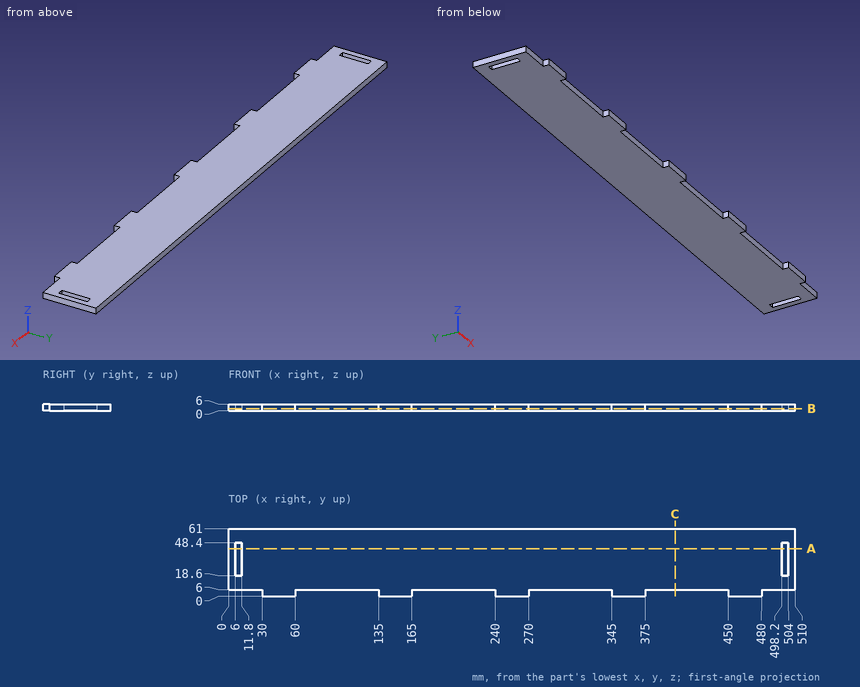
Could you check a few things on this drawing? It's one solid part, dimensions in mm from its lowest x, y, z. Round coordinates to 2 decimals unless told otherwise and drop trailing zeros. Loops run counter-clockwise (first coordinate to the right, second up) from the corner with the lowest first, then second, coordinate; pieces in that order, holes last. Notation, with made-up numbers: (16, -34.5) -> (47, -34.5) arc R28 cw to (47, -6.5) -> close; hole circle Ø1 at (45.5, 68.5). An arc over 180 degrees is marked (long way). One line per item, written item: value. Start each with the question number.
1. If we section it at B-B, the plane z = 1.75: Give the number of separate pieces and of enclosed holes in the cut face, then the cut area to 3 significant figures.
2. If I drill on probe 1 along X at (y, z) = (30, 2.5); probe 2 along Y at (x, z) = (306, 2.65), over which ranges is the centre line in solid material (lowest first)?
3. If we section it at A-A, the plane y = 43: Write out the boundary of the cut face in (x, z).
4. For pin 1 (3 mm diameter, centred on y = 3, z = 3.5, fed in from -X); pin 2 (3 mm diameter, centred on y = 3, z = 2.5, fed in from +X); pin 3 (3 mm diameter, centred on x = 7.5, z = 3, fed in from -Y), each with a flat end and sliding along its axis, tell me the tip position at first contact or that it passes through.
5. If we section it at C-C, the plane x = 402: Write out the boundary of the cut face in (y, z).
Calculated:
1. separate pieces: 1
1. enclosed holes: 2
1. area: 28,600 mm²
2. probe 1: x = 0 to 6, 11.8 to 498.2, 504 to 510
2. probe 2: y = 6 to 61
3. outline: (0, 0) -> (6, 0) -> (6, 6) -> (0, 6) -> close; (11.8, 0) -> (498.2, 0) -> (498.2, 6) -> (11.8, 6) -> close; (504, 0) -> (510, 0) -> (510, 6) -> (504, 6) -> close
4. pin 1: stops at x = 30
4. pin 2: stops at x = 480
4. pin 3: stops at y = 6
5. outline: (6, 0) -> (61, 0) -> (61, 6) -> (6, 6) -> close
